Autodesk Inventor part; units mm, degrees
ref_plane "Work Plane1" through (0, 0, -155) normal (0, 0, -1) x (-1, 0, 0)
ref_plane "YZ Plane" through (0, 0, 0) normal (1, 0, 0) x (0, 1, 0)
ref_plane "XZ Plane" through (0, 0, 0) normal (0, 1, 0) x (-1, 0, 0)
sketch "Sketch1" plane through (0, 0, 0) normal (0, 0, 1) x (1, 0, 0)
  circle A0 centre (0, 0) radius 4
  dimension "d0" = 8
extrude "Extrusion1" add sketch "Sketch1" against normal blind 310
sketch "Sketch2" plane through (0, 0, 0) normal (0, 0, 1) x (1, 0, 0)
  line L0 (-10, 10) -> (10, 10)
  line L1 (10, 10) -> (10, -10)
  line L2 (10, -10) -> (-10, -10)
  line L3 (-10, -10) -> (-10, 10)
  line L4 (-10, 10) -> (10, -10) construction
  line L5 (10, 10) -> (-10, -10) construction
  point P0 (0, 0)
  dimension "d3" = 20
extrude "Extrusion2" add sketch "Sketch2" along normal blind 5
ref_plane "Work Plane1" through (0, 0, -155) normal (0, 0, -1) x (-1, 0, 0)
mirror "Mirror1" about plane through (0, 0, -155) normal (0, 0, -1) of "Extrusion2"
properties part number "front axle" material "Steel, Mild"
Can you work these out from the model? Positions are in its coordinate system, mm. A direction names the side the tool comes from. Coordinates: 2 decimals unless noted, no trailing zeros. Loops run counter-clockwise (first coordinate to the right, second up) from the corner with the lowest first, then second, coordinate; pieces in that order, holes last. Notation, with made-up numbers: M -11.75,22 L 23.25,22 A22 ccw 23.25,31 Z; hole C 53.25,76 d3. An arc over 180 degrees is marked long. Answer as CSV lines item,"result". Start each with the question number.
1. For faces 1 (the face through (4.3, 0.1, 0)), 2 (the face through (10, 0, 2)), which set-ups out of +Z, -Z, +X, -X, +Y, -Y let a thin tool reach every point of the face, with its end or its side?
2. If I drill on probe 1 along Z at (x, y) = (3, -6.75); probe 2 along X at (y, z) = (-0.5, -190.5), over which ranges is the centre line in solid material (lowest first)? Write a range as [from, to].
3. Suppose I cut it at C-C, the plane z = -115.5. List the corners of the cut face in (x, y) for me, plus the area to 3 significant figures.
4. For pin 1 Ø1 at (x, z) = (-1.5, -137) entering from +Y; pin 2 Ø4 at (y, z) = (-1.5, -101.5) entering from -X; pin 3 Ø12 at (y, z) = (-4, -182.5) entering from +X, each with a flat end and sliding along its axis, tell me the tip position at first contact or that it passes through.
5. Suppose I cut it at B-B, the plane x = 0. List the corners of the cut face in (y, z) for me.
6. Suppose I cut it at A-A, the plane y = -6.75. List the corners of the cut face in (x, z) for me.
7. Thinking about a two-plate mould opening in Z: for faces 3 (the face through (0, -10, 2)), 4 (the face through (0, 0, 5)), 5 (the face through (-4.3, 0.1, -310)), which applies, +Z half, -Z half, draft (parallel to the pull), parting line (faces both ways), or undercut?
Output:
1,face 1,"none"
1,face 2,"+Z, -Z, +X, +Y, -Y"
2,probe 1,"z = [-315, -310], [0, 5]"
2,probe 2,"x = [-3.97, 3.97]"
3,outline,"C 0,0 d8"
3,area,"50.3 mm^2"
4,pin 1,"stops at y = 3.87"
4,pin 2,"stops at x = -4"
4,pin 3,"stops at x = 4"
5,outline,"M -10,-315 L 10,-315 L 10,-310 L 4,-310 L 4,0 L 10,0 L 10,5 L -10,5 L -10,0 L -4,0 L -4,-310 L -10,-310 Z"
6,outline,"M -10,-315 L 10,-315 L 10,-310 L -10,-310 Z; M -10,0 L 10,0 L 10,5 L -10,5 Z"
7,face 3,"draft"
7,face 4,"+Z half"
7,face 5,"undercut"
